Read the model definition and answer for the solid it produces. Units are mm, in the model's axes. A direction names the side the tool comes from. Coordinates: 2 decimals unless noted, no trailing zeros. Write each loop counter-clockwise with the first axis right and the second up, starting at its lowest first coordinate (ties: lowest second). Pieces come first, ordered by that corner, then holes.
1) Determine the mould class of faces 1 (the face through (0, -1, 325)), 2 (the face through (-0.61, -3.62, 322.75)), 3 (the face through (0, -4, 324)) for opening direction Z: +Z half, -Z half, draft (parallel to the pull), parting line (faces both ways), or undercut.
2) The part is cut by section A-A (y = -1.75). Determine the outline of the cut face in (x, z).
3) The part is cut by section B-B (x = 0.75). Determine the outline of the cut face in (y, z), then the cut area to 3 significant figures.
4) Find the intervals of material crossed by line 1 (Z direction, x = -1.25, y = -3.5); line 2 (Y direction, x = -0.5, z = 239.5); line 3 (Z direction, x = -0.5, y = 3.5), in increasing order.
5) Which of the six approach directions +Z, -Z, +X, -X, +Y, -Y give full straight-line access (tool end or side, diameter ignored) to faces 4 (the face through (0, 0, 25)), 5 (the face through (0, 2.5, 321)), 6 (the face through (-0.1, -3.5, 323.3))?
6) Each of these flat-tipped pins is pushed along its axis until it touches: pin 1 Ø1.9 at (x, z) = (-1, 321) entering from +Y; pin 2 Ø1.5 at (x, z) = (1.5, 80.5) entering from +Y. Where does it stop, or does it pass through?
7) The part is cut by section C-C (z = 57). Determine the outline of the cut face in (x, y), then the cut area to 3 significant figures.
from build123d import *

# Parameters (mm, degrees)
SKETCH1_R           = 4
BOSS_EXTRUDE1_DEPTH = 325
CUT_EXTRUDE1_DEPTH  = 7.5
SKETCH3_R           = 4
SKETCH3_R_2         = 3.5
CUT_EXTRUDE2_DEPTH  = 1
SKETCH5_R           = 4
CUT_EXTRUDE3_DEPTH  = 65
SKETCH6_R           = 4
BOSS_EXTRUDE2_DEPTH = 13
SKETCH7_R           = 4
BOSS_EXTRUDE3_DEPTH = 10
SKETCH8_R           = 4
BOSS_EXTRUDE4_DEPTH = 40
SKETCH9_R           = 4
CUT_EXTRUDE4_DEPTH  = 30
SKETCH10_R          = 4
CUT_EXTRUDE5_DEPTH  = 61
SKETCH11_R          = 4
BOSS_EXTRUDE5_DEPTH = 68


with BuildPart() as part:
    # Sketch1 → Boss-Extrude1 (new body)
    with BuildSketch(Plane.XY):
        Circle(SKETCH1_R)
    extrude(amount=BOSS_EXTRUDE1_DEPTH)

    # Sketch2 → Cut-Extrude1 (cut)
    with BuildSketch(Plane.XY.offset(325)):
        with BuildLine():
            Line((3.122498999, 2.5), (-3.122498999, 2.5))
            ThreePointArc((-3.122498999, 2.5), (0, 4), (3.122498999, 2.5))
        make_face()
    extrude(amount=-CUT_EXTRUDE1_DEPTH, mode=Mode.SUBTRACT)

    # Sketch3 → Cut-Extrude2 (cut)
    with BuildSketch(Plane.XY.offset(323.75)):
        Circle(SKETCH3_R)
        Circle(SKETCH3_R_2, mode=Mode.SUBTRACT)
    extrude(amount=-CUT_EXTRUDE2_DEPTH, mode=Mode.SUBTRACT)

    # Sketch5 → Cut-Extrude3 (cut)
    with BuildSketch(Plane(origin=(0, 0, 0), x_dir=(-1, 0, 0), z_dir=(0, 0, -1))):
        Circle(SKETCH5_R)
    extrude(amount=-CUT_EXTRUDE3_DEPTH, mode=Mode.SUBTRACT)

    # Sketch6 → Boss-Extrude2 (add)
    with BuildSketch(Plane(origin=(0, 0, 65), x_dir=(-1, 0, 0), z_dir=(0, 0, -1))):
        Circle(SKETCH6_R)
    extrude(amount=BOSS_EXTRUDE2_DEPTH)

    # Sketch7 → Boss-Extrude3 (add)
    with BuildSketch(Plane(origin=(0, 0, 52), x_dir=(-1, 0, 0), z_dir=(0, 0, -1))):
        Circle(SKETCH7_R)
    extrude(amount=BOSS_EXTRUDE3_DEPTH)

    # Sketch8 → Boss-Extrude4 (add)
    with BuildSketch(Plane(origin=(0, 0, 42), x_dir=(-1, 0, 0), z_dir=(0, 0, -1))):
        Circle(SKETCH8_R)
    extrude(amount=BOSS_EXTRUDE4_DEPTH)

    # Sketch9 → Cut-Extrude4 (cut)
    with BuildSketch(Plane(origin=(0, 0, 2), x_dir=(-1, 0, 0), z_dir=(0, 0, -1))):
        Circle(SKETCH9_R)
    extrude(amount=-CUT_EXTRUDE4_DEPTH, mode=Mode.SUBTRACT)

    # Sketch10 → Cut-Extrude5 (cut)
    with BuildSketch(Plane(origin=(0, 0, 32), x_dir=(-1, 0, 0), z_dir=(0, 0, -1))):
        Circle(SKETCH10_R)
    extrude(amount=-CUT_EXTRUDE5_DEPTH, mode=Mode.SUBTRACT)

    # Sketch11 → Boss-Extrude5 (add)
    with BuildSketch(Plane(origin=(0, 0, 93), x_dir=(-1, 0, 0), z_dir=(0, 0, -1))):
        Circle(SKETCH11_R)
    extrude(amount=BOSS_EXTRUDE5_DEPTH)


solid = part.part
Reported:
1. face 1: +Z half
1. face 2: undercut
1. face 3: draft
2. outline: (-3.6, 25) - (3.6, 25) - (3.6, 322.75) - (3.03, 322.75) - (3.03, 323.75) - (3.6, 323.75) - (3.6, 325) - (-3.6, 325) - (-3.6, 323.75) - (-3.03, 323.75) - (-3.03, 322.75) - (-3.6, 322.75) - close
3. outline: (-3.93, 25) - (3.93, 25) - (3.93, 317.5) - (2.5, 317.5) - (2.5, 325) - (-3.93, 325) - (-3.93, 323.75) - (-3.42, 323.75) - (-3.42, 322.75) - (-3.93, 322.75) - close
3. area: 2,350 mm2
4. line 1: z = 25 to 322.75, 323.75 to 325
4. line 2: y = -3.97 to 3.97
4. line 3: z = 25 to 317.5
5. face 4: -Z, +X, -X, +Y, -Y
5. face 5: +Z, +X, -X, +Y
5. face 6: none
6. pin 1: stops at y = 2.5
6. pin 2: stops at y = 3.93
7. outline: circle Ø8 at (0, 0)
7. area: 50.3 mm2
